Check sheet for the modelled part. Datum: model origin and axes. Units: mm. Coordinates: 2 decimals unless noted, no trailing zeros. Loops run counter-clockwise (first coordinate to the right, second up) from the corner with the lowest first, then second, coordinate; pieces in that order, holes last. Notation, with made-up numbers: (88.5, -38.75) -> (98.5, -38.75) arc R26 cw to (98.5, -9.75) -> close; hole circle Ø7 at (24, 47.25). An arc over 180 degrees is marked (long way). Use CSV: the item, a comma, the result in double quotes. Start each with the question number.
1. Sectioned sample at C-C, the plane x = -55.5. Record the cut outline in (y, z).
2. Sectioned sample at A-A, the plane z = 8.75. Record the cut outline in (x, y), and give its area (3 significant figures).
3. Sectioned sample at B-B, the plane x = 52. Record the cut outline in (y, z), and give its area (3 significant figures).
4. Thickness scan on L1, parallel to Y at x = -88.9, z = 7.5; L2, parallel to Y at x = -38.5, z = 4.5; L3, parallel to Y at x = -52, z = 11. Record the ranges inside material, lowest first.
5. Gauge pin test, flat ends, axial feed: pin 1 (5.5 mm diameter, centred on x = -88.9, y = -325.72, fed in from +Z); pin 2 (2 mm diameter, centred on x = -44.5, z = 7, fed in from -Y). Record the tip position at first contact, or that the pin passes through.
```python
from build123d import *

# Parameters (mm, degrees)
F0_R     = 1.7272
F1_DEPTH = 12.7


with BuildPart() as f1:
    # F0 (on Top) → F1 (new body)
    with BuildSketch(Plane.XY):
        with BuildLine():
            Line((101.6, -325.721193), (101.6, 325.721193))
            ThreePointArc((101.6, 325.721193), (99.77563, 332.279444), (94.826667, 336.953495))
            ThreePointArc((94.826667, 336.953495), (0, 360.436653), (-94.826667, 336.953495))
            ThreePointArc((-94.826667, 336.953495), (-99.77563, 332.279444), (-101.6, 325.721193))
            Line((-101.6, 325.721193), (-101.6, -325.721193))
            ThreePointArc((-101.6, -325.721193), (-99.77563, -332.279444), (-94.826667, -336.953495))
            ThreePointArc((-94.826667, -336.953495), (0, -360.436653), (94.826667, -336.953495))
            ThreePointArc((94.826667, -336.953495), (99.77563, -332.279444), (101.6, -325.721193))
        make_face()
        with Locations((-88.9, -325.721193)):
            Circle(F0_R, mode=Mode.SUBTRACT)
        with Locations((0, -347.736653)):
            Circle(F0_R, mode=Mode.SUBTRACT)
        with Locations((88.9, -325.721193)):
            Circle(F0_R, mode=Mode.SUBTRACT)
        with Locations((-88.9, 325.721193)):
            Circle(F0_R, mode=Mode.SUBTRACT)
        with Locations((0, 347.736653)):
            Circle(F0_R, mode=Mode.SUBTRACT)
        with Locations((88.9, 325.721193)):
            Circle(F0_R, mode=Mode.SUBTRACT)
    extrude(amount=F1_DEPTH)


solid = f1.part
```
Completed:
1,outline,"(-352.71, 0) -> (352.71, 0) -> (352.71, 12.7) -> (-352.71, 12.7) -> close"
2,outline,"(-101.6, -325.72) arc R12.7 ccw to (-94.83, -336.95) arc R203.2 ccw to (94.83, -336.95) arc R12.7 ccw to (101.6, -325.72) -> (101.6, 325.72) arc R12.7 ccw to (94.83, 336.95) arc R203.2 ccw to (-94.83, 336.95) arc R12.7 ccw to (-101.6, 325.72) -> close; hole circle Ø3.45 at (-88.9, -325.72); hole circle Ø3.45 at (-88.9, 325.72); hole circle Ø3.45 at (0, -347.74); hole circle Ø3.45 at (0, 347.74); hole circle Ø3.45 at (88.9, -325.72); hole circle Ø3.45 at (88.9, 325.72)"
2,area,"143,000 mm²"
3,outline,"(-353.67, 0) -> (353.67, 0) -> (353.67, 12.7) -> (-353.67, 12.7) -> close"
3,area,"8,980 mm²"
4,L1,"-339.96 to -327.45, -323.99 to 323.99, 327.45 to 339.96"
4,L2,"-356.76 to 356.76"
4,L3,"-353.67 to 353.67"
5,pin 1,"z = 12.7"
5,pin 2,"y = -355.73"
